Source: CAD feature listing. Evaluate the final solid. Frame: model axes, mm. Face numbers are marked on the shaded views. A direction names the side the tool comes from. Give positions to 0.01 mm unless a question says otherwise; leave off trailing zeros. Order: outer loops, then holes, each group sorted by start corner. A loop starts at its lowest first (then second) coordinate and runs counter-clockwise, first axis right, second up.
from build123d import *

# Parameters (mm, degrees)
SKETCH1_R           = 12.5
SKETCH1_R_2         = 3
BOSS_EXTRUDE1_DEPTH = 25
SKETCH2_R           = 7
CUT_EXTRUDE1_DEPTH  = 12.5
SKETCH3_R           = 1.65
CUT_EXTRUDE2_DEPTH  = 31.618621785


with BuildPart() as part:
    # Sketch1 → Boss-Extrude1 (new body)
    with BuildSketch(Plane(origin=(0, 0, 0), x_dir=(1, 0, 0), z_dir=(0, 1, 0))):
        with Locations(Location((0, 0, 0), (0, 0, 270))):
            Circle(SKETCH1_R)
        with Locations(Location((0, 0, 0), (0, 0, 270))):
            Circle(SKETCH1_R_2, mode=Mode.SUBTRACT)
    extrude(amount=BOSS_EXTRUDE1_DEPTH)

    # Sketch2 → Cut-Extrude1 (cut)
    with BuildSketch(Plane(origin=(0, 25, 0), x_dir=(1, 0, 0), z_dir=(0, 1, 0))):
        with Locations(Location((0, 0, 0), (0, 0, 270))):
            Circle(SKETCH2_R)
    extrude(amount=-CUT_EXTRUDE1_DEPTH, mode=Mode.SUBTRACT)

    # Sketch3 → Cut-Extrude2 (cut, through all)
    with BuildSketch(Plane.XY):
        with Locations(Location((0, 5, 0), (0, 0, 90.000000006))):
            Circle(SKETCH3_R)
        with Locations(Location((0, 20, 0), (0, 0, 90))):
            Circle(SKETCH3_R)
    extrude(amount=CUT_EXTRUDE2_DEPTH, mode=Mode.SUBTRACT)


solid = part.part
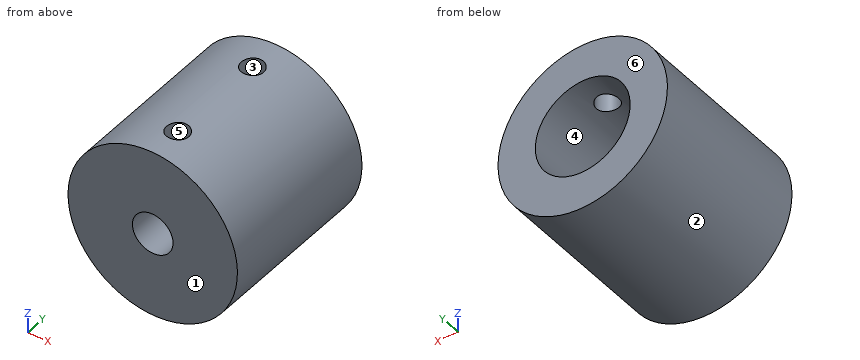
1) Section query A-A on z = 0. Output: boundary loops of the cut face in (x, y), and give its area (3 significant figures).
Checks:
outline: (-12.5, 0) - (-3, 0) - (-3, 12.5) - (-7, 12.5) - (-7, 25) - (-12.5, 25) - close; (3, 0) - (12.5, 0) - (12.5, 25) - (7, 25) - (7, 12.5) - (3, 12.5) - close
area: 375 mm2
2) Section query D-D on z = 5.75. Output: boundary loops of the cut face in (x, y).
Checks:
outline: (-11.1, 0) - (11.1, 0) - (11.1, 25) - (3.99, 25) - (3.99, 12.5) - (-3.99, 12.5) - (-3.99, 25) - (-11.1, 25) - close; hole circle Ø3.3 at (0, 5)
3) Reachability of the marked faces 5 and 6 from +Z, -Z, +X, -X, +Y, -Y: full face, straight path, thin tool, end or side. Return the list, or none.
Checks:
face 5: +Z
face 6: +Z, -Z, +X, -X, +Y
4) Section query B-B on x = 0. Output: boundary loops of the cut face in (y, z).
Checks:
outline: (0, -12.5) - (25, -12.5) - (25, -7) - (12.5, -7) - (12.5, -3) - (0, -3) - close; (0, 3) - (3.35, 3) - (3.35, 12.5) - (0, 12.5) - close; (6.65, 3) - (12.5, 3) - (12.5, 7) - (18.35, 7) - (18.35, 12.5) - (6.65, 12.5) - close; (21.65, 7) - (25, 7) - (25, 12.5) - (21.65, 12.5) - close
5) Ray query, L1, parallel to Y at x = 0, z = 10.95; L2, parallel to Y at x = 0, z = 5.25; L3, parallel to X at y = 20.5, z = 3.75. Return the intervals inside material, ascending.
Checks:
L1: y = 0 to 3.35, 6.65 to 18.35, 21.65 to 25
L2: y = 0 to 3.35, 6.65 to 12.5
L3: x = -11.92 to -5.91, 5.91 to 11.92
6) Pull-direction query (X, two-part tool) for the marked faces 1, 2, 3 and 4; classes: +X half, -X half, draft (parallel to the pull), parting line (faces both ways), or undercut.
Checks:
face 1: draft
face 2: parting line
face 3: undercut
face 4: undercut
7) Section query C-C on y = 17.75. Output: boundary loops of the cut face in (x, z).
Checks:
outline: circle Ø25 at (0, 0); hole circle Ø14 at (0, 0)
8) First-contact query: pin 1 Ø2 at (x, y) = (-8.5, 17) entering from +Z; pin 2 Ø5 at (x, z) = (0, 0) entering from -Y; pin 3 Ø10 at (y, z) = (10.5, -9.5) entering from +X; pin 4 Ø1 at (x, y) = (1.5, 15.5) entering from +Z. Flat tips, straight axial feed; report the tip coordinate or a pass-through.
Checks:
pin 1: stops at z = 10
pin 2: passes through
pin 3: stops at x = 11.66
pin 4: stops at z = 12.46
